from build123d import *

# Parameters (mm, degrees)
F0_R     = 20
F0_R_2   = 17.25
F1_DEPTH = 1.5
F2_R     = 20
F2_R_2   = 18.25
F3_DEPTH = 1
F4_R     = 20
F4_R_2   = 17.25
F5_DEPTH = 15
F6_R     = 1.3
F7_SIZE  = 0.99999


# Not quite as in the source:
# - a fillet or chamfer is up to 0.001 mm smaller than in the source, because OpenCascade refuses the exact size


with BuildPart() as f1:
    # F0 (on Top) → F1 (new body)
    with BuildSketch(Plane.XY):
        Circle(F0_R)
        Circle(F0_R_2, mode=Mode.SUBTRACT)
    extrude(amount=F1_DEPTH)

    # F2 (on face) → F3 (join)
    with BuildSketch(Plane.XY.offset(1.5)):
        Circle(F2_R)
        Circle(F2_R_2, mode=Mode.SUBTRACT)
    extrude(amount=F3_DEPTH)

    # F4 (on face) → F5 (join)
    with BuildSketch(Plane.XY.offset(2.5)):
        Circle(F4_R)
        Circle(F4_R_2, mode=Mode.SUBTRACT)
    extrude(amount=F5_DEPTH)

    # F6
    f6_edges = [f1.edges().sort_by_distance(p)[0] for p in [
        (-17.25, 0, 17.5),
        (-20, 0, 17.5),
    ]]
    fillet(f6_edges, radius=F6_R)

    # F7 (size 1 in the source; OpenCascade refuses exactly that, so slightly less here)
    f7_edges = [f1.edges().sort_by_distance(p)[0] for p in [
        (-17.25, 0, 2.5),
    ]]
    chamfer(f7_edges, length=F7_SIZE)


solid = f1.part
CAD build for the part. Positions are in the model's coordinates, mm. A direction names the side the tool comes from. Coordinates: 2 decimals unless noted, no trailing zeros. Write each loop counter-clockwise with the first axis right and the second up, starting at its lowest first coordinate (ties: lowest second). Pieces come first, ordered by that corner, then holes. Notation, with made-up numbers: M 78.5,-35.5 L 92.5,-35.5 A18 ccw 92.5,-21.5 Z; hole C 52,84 d4. An arc over 180 degrees is marked long. Return JSON: item names as keys, results as strings.
Item 1: Two-plate mould, pull along Y, no slides. Class faces 1 (the flat face through (-15, -9, 0)), 2 (the cylindrical face through (-4.336, -19.524, 7.987)), 3 (the cylindrical face through (-3.956, -17.816, 1.993)): +Y half, -Y half, draft (parallel to the pull), parting line (faces both ways), or undercut.
Findings below:
{"face 1": "draft", "face 2": "parting line", "face 3": "undercut"}
Item 2: Which spindle directions (+Z, -Z, +X, -X, +Y, -Y) get a long thin tool onto all of the face, cutting with end or side? Do faces 4 (the cylindrical face through (16.453, 5.181, 0.74)), 5 (the flat face through (7, -16, 1.5)). Say none if no direction does.
Findings below:
{"face 4": "+Z, -Z", "face 5": "none"}
Item 3: Slice it at C-C, the plane z = 14. Write the cut outline in (x, y), and give its area (3 significant figures).
Findings below:
{"outline": "C 0,0 d40; hole C 0,0 d34.5", "area": "322 mm2"}
Item 4: Probe line 1 (Y direction, x = 0, z = 2.15); line 2 (Y direction, x = 0, z = 6.75); line 3 (X direction, y = -11, z = 13.25). List the from-to ranges inside material, lowest first. Write a range as from..to.
Findings below:
{"line 1": "y = -20..-18.25, 18.25..20", "line 2": "y = -20..-17.25, 17.25..20", "line 3": "x = -16.7..-13.29, 13.29..16.7"}
Item 5: Drop flat-ended pins along their axis: pin 1 Ø6 at (y, z) = (-5, 7.5) entering from -X; pin 2 Ø4 at (x, z) = (2, 3) entering from +Y; pin 3 Ø1 at (x, z) = (-3.5, 3) entering from +Y. Give the stop position or say it passes through.
Findings below:
{"pin 1": "stops at x = -19.9", "pin 2": "stops at y = 20", "pin 3": "stops at y = 19.77"}
